```python
from build123d import *

# Parameters (mm, degrees)
BOSS_EXTRUDE1_DEPTH = 200
BOSS_EXTRUDE2_START = -11.5
SKETCH2_R           = 8.1
BOSS_EXTRUDE2_DEPTH = 7
BOSS_EXTRUDE3_START = -18.5
SKETCH3_W           = 10
SKETCH3_H           = 10
SKETCH3_R           = 1.75
BOSS_EXTRUDE3_DEPTH = 7
FILLET1_R           = 5
SKETCH5_R           = 1.5
CUT_EXTRUDE1_DEPTH  = 7


with BuildPart() as part:
    # Sketch1 → Boss-Extrude1 (new body)
    with BuildSketch(Plane.XY):
        Polygon((25, 20), (30, 20), (30, 0), (0, 0), (0, 20), (5, 20), (5, 5), (25, 5), align=None)
    extrude(amount=BOSS_EXTRUDE1_DEPTH)

    # Sketch2 → Boss-Extrude2 (add)
    with BuildSketch(Plane(origin=(30, 0, 0), x_dir=(0, 0, -1), z_dir=(1, 0, 0)).offset(BOSS_EXTRUDE2_START)):
        with BuildLine():
            Line((-115, -15), (-115, -10))
            ThreePointArc((-115, -10), (-117.928932188, -2.928932188), (-125, 0))
            Line((-125, 0), (-75, 0))
            ThreePointArc((-75, 0), (-82.071067812, -2.928932188), (-85, -10))
            Line((-85, -10), (-85, -15))
            ThreePointArc((-85, -15), (-100, -30), (-115, -15))
        make_face()
        with Locations(Location((-100, -15, 0), (0, 0, 90))):
            Circle(SKETCH2_R, mode=Mode.SUBTRACT)
    extrude(amount=-BOSS_EXTRUDE2_DEPTH)

    # Sketch3 → Boss-Extrude3 (add)
    with BuildSketch(Plane(origin=(30, 0, 0), x_dir=(0, 0, -1), z_dir=(1, 0, 0)).offset(BOSS_EXTRUDE3_START)):
        with Locations((-195, -5)):
            Rectangle(SKETCH3_W, SKETCH3_H)
        with Locations(Location((-195, -5, 0), (0, 0, 90))):
            Circle(SKETCH3_R, mode=Mode.SUBTRACT)
    extrude(amount=BOSS_EXTRUDE3_DEPTH)

    # Fillet1
    fillet1_edges = [part.edges().sort_by_distance(p)[0] for p in [
        (15, -10, 190),
        (15, -10, 200),
    ]]
    fillet(fillet1_edges, radius=FILLET1_R - 0.0001)  # a hair under: the kernel refuses the full size

    # Sketch5 → Cut-Extrude1 (cut)
    with BuildSketch(Plane(origin=(0, 5, 0), x_dir=(1, 0, 0), z_dir=(0, 1, 0))):
        with Locations(Location((15, -180, 0), (0, 0, 270))):
            Circle(SKETCH5_R)
        with Locations(Location((15, -160, 0), (0, 0, 270))):
            Circle(SKETCH5_R)
        with Locations(Location((15, -40, 0), (0, 0, 270))):
            Circle(SKETCH5_R)
        with Locations(Location((15, -20, 0), (0, 0, 270))):
            Circle(SKETCH5_R)
    extrude(amount=-CUT_EXTRUDE1_DEPTH, mode=Mode.SUBTRACT)


solid = part.part
```
Read the model definition and answer for the solid it produces. Units are mm, in the model's axes. A direction names the side the tool comes from. Give positions to 0.01 mm unless a question says otherwise; leave off trailing zeros. Write each loop counter-clockwise with the first axis right and the second up, starting at its lowest first coordinate (ties: lowest second). Pieces come first, ordered by that corner, then holes. Notation, with made-up numbers: (-12, 88.5) - (28, 88.5) arc R9 ccw to (28, 101.5) - close; hole circle Ø10 at (2, 70). An arc over 180 degrees is marked (long way). Write item = value, one per line. Start each with the question number.
Item 1: Find the intervals of material crossed by probe 1 along X at (y, z) = (13, 36); probe 2 along X at (y, z) = (3, 40); probe 3 along Z at (x, y) = (16.5, -5), in increasing order. Write a range as [from, to].
Item 2: Find section D-D (x = 27). Give the vertices of the cut face in (y, z), then the cut area to 3 significant figures.
Item 3: The mould has two halves that part along Z. Classify faces 5 (the cylindrical face through (15, -30, 100)), 6 (the flat face through (19, 3, 0)), 7 (the cylindrical face through (15, -8, 191)), 8 (the flat face through (11.5, -8, 105)): +Z half, -Z half, draft (parallel to the pull), parting line (faces both ways), or undercut.
Item 4: Each of these flat-tipped pins is pushed along its axis until it touches: P1, Ø10, axis at x = 12.5, z = 89.5, coming from the +Y side; P2, Ø9, axis at x = 16, z = 113.5, coming from the -Y side; P3, Ø5.5, axis at x = 16.5, y = -13.5, coming from the +Z side. Where does it stop, or does it pass through?
Item 5: Find section B-B (z = 13). Give the vertices of the cut face in (x, y).
Item 6: A tool of negligible diameter and unlimited length cuts with its end or side. For faces 1 (the flat face through (11.5, -3, 195)), 2 (the flat face through (18.5, -8, 105)), 3 (the flat face through (5, 13, 99)), 4 (the flat face through (15, -3, 190)), from which of +Z, -Z, +X, -X, +Y, -Y can it reach the whole face along a straight path? Write none if from no direction.
Item 7: Find section A-A (z = 100). Give the vertices of the cut face in (x, y), then the cut area to 3 significant figures.
Item 8: Find section C-C (y = -19.5). Give the vertices of the cut face in (x, z), then the cut area to 3 significant figures.
Response:
q1.probe_1 = [0, 5], [25, 30]
q1.probe_2 = [0, 13.5], [16.5, 30]
q1.probe_3 = [83.66, 116.34], [190, 193.25], [196.75, 200]
q2.outline = (0, 0) - (20, 0) - (20, 200) - (0, 200) - close
q2.area = 4,000 mm²
q3.face_5 = parting line
q3.face_6 = -Z half
q3.face_7 = undercut
q3.face_8 = draft
q4.P1 = 5
q4.P2 = -27
q4.P3 = 115
q5.outline = (0, 0) - (30, 0) - (30, 20) - (25, 20) - (25, 5) - (5, 5) - (5, 20) - (0, 20) - close
q6.face_1 = +Z, -Z, -X, -Y
q6.face_2 = +Z, -Z, +X, -Y
q6.face_3 = +Z, -Z, +Y
q6.face_4 = +X, -X, -Y
q7.outline = (0, 0) - (11.5, 0) - (11.5, -6.9) - (18.5, -6.9) - (18.5, 0) - (30, 0) - (30, 20) - (25, 20) - (25, 5) - (5, 5) - (5, 20) - (0, 20) - close; (11.5, -30) - (18.5, -30) - (18.5, -23.1) - (11.5, -23.1) - close
q7.area = 397 mm²
q8.outline = (11.5, 85.69) - (18.5, 85.69) - (18.5, 93.27) - (11.5, 93.27) - close; (11.5, 106.73) - (18.5, 106.73) - (18.5, 114.31) - (11.5, 114.31) - close
q8.area = 106 mm²
